```python
from build123d import *

# Parameters (mm, degrees)
SKETCH1_R           = 1.499997
SKETCH1_R_2         = 5.08
BOSS_EXTRUDE1_DEPTH = 13.97
CUT_EXTRUDE1_DEPTH  = 3
FILLET1_R           = 1.27
SKETCH3_R           = 3.302
CUT_EXTRUDE2_DEPTH  = 41.275
CUT_EXTRUDE3_DEPTH  = 5.842
BOSS_EXTRUDE2_DEPTH = 25.4
FILLET2_R           = 2.54


with BuildPart() as part:
    # Sketch1 → Boss-Extrude1 (new body)
    with BuildSketch(Plane.XY):
        Polygon((-12.7, 33.2994), (-5.715, 33.2994), (-5.715, 39.6494), (5.715, 39.6494), (5.715, 33.2994), (28.575, 33.2994), (28.575, -33.2994), (5.715, -33.2994), (5.715, -39.6494), (-5.715, -39.6494), (-5.715, -33.2994), (-12.7, -33.2994), align=None)
        with Locations((0, 8.001)):
            Circle(SKETCH1_R, mode=Mode.SUBTRACT)
        with Locations((8.001, 0)):
            Circle(SKETCH1_R, mode=Mode.SUBTRACT)
        Circle(SKETCH1_R_2, mode=Mode.SUBTRACT)
        with Locations((0, -8.001)):
            Circle(SKETCH1_R, mode=Mode.SUBTRACT)
        with Locations((-8.001, 0)):
            Circle(SKETCH1_R, mode=Mode.SUBTRACT)
    extrude(amount=BOSS_EXTRUDE1_DEPTH)

    # Sketch2 → Cut-Extrude1 (cut)
    with BuildSketch(Plane(origin=(0, 0, 0), x_dir=(-1, 0, 0), z_dir=(0, 0, -1))):
        Polygon((8.001, -3.579571669), (11.101, -1.789785834), (11.101, 1.789785834), (8.001, 3.579571669), (4.901, 1.789785834), (4.901, -1.789785834), align=None)
        Polygon((3.579571669, 8.001), (1.789785834, 11.101), (-1.789785834, 11.101), (-3.579571669, 8.001), (-1.789785834, 4.901), (1.789785834, 4.901), align=None)
        Polygon((-3.579571669, -8.001), (-1.789785834, -11.101), (1.789785834, -11.101), (3.579571669, -8.001), (1.789785834, -4.901), (-1.789785834, -4.901), align=None)
        Polygon((-8.001, 3.579571669), (-11.101, 1.789785834), (-11.101, -1.789785834), (-8.001, -3.579571669), (-4.901, -1.789785834), (-4.901, 1.789785834), align=None)
    extrude(amount=-CUT_EXTRUDE1_DEPTH, mode=Mode.SUBTRACT)

    # Fillet1
    # the kernel refuses this fillet: 1.27 mm, written as the material it takes off along each edge
    with BuildSketch(Plane(origin=(-4.901, -1.336637198, 3), x_dir=(0.3505491054701989, -0.9365443527425935, 0), z_dir=(0, 0, -1)), Plane(origin=(-1.336637198, 4.901, 3), x_dir=(-0.9365443527425947, -0.3505491054701953, 0), z_dir=(0, 0, -1)), Plane(origin=(1.336637198, -4.901, 3), x_dir=(0.9365443527425922, 0.3505491054702024, 0), z_dir=(0, 0, -1))) as fillet1_piece_1:
        with BuildLine():
            CenterArc((1.048997579, 1.264640212), FILLET1_R, 240.540119445, 24.194103812)
            Line((0.424393796, 0.158850849), (0, 0))
            ThreePointArc((0, 0), (0.466221146, 0.021439153), (0.932442292, 0))
        make_face()
    extrude(amount=5.331105731, mode=Mode.SUBTRACT)
    with BuildSketch(Plane(origin=(-4.901, 1.336637198, 3), x_dir=(0.35054910547019297, 0.9365443527425957, 0), z_dir=(0, 0, -1)), Plane(origin=(1.336637198, 4.901, 3), x_dir=(0.9365443527425946, -0.3505491054701959, 0), z_dir=(0, 0, -1)), Plane(origin=(-1.336637198, -4.901, 3), x_dir=(-0.9365443527425968, 0.35054910547018975, 0), z_dir=(0, 0, -1))) as fillet1_piece_2:
        with BuildLine():
            CenterArc((1.048997579, -1.264640212), FILLET1_R, 95.265776743, 24.194103812)
            Line((0.424393796, -0.158850849), (0, 0))
            ThreePointArc((0, 0), (0.466221146, -0.021439153), (0.932442292, 0))
        make_face()
    extrude(amount=5.331105731, mode=Mode.SUBTRACT)
    with BuildSketch(Plane(origin=(4.901, 1.336637198, 3), x_dir=(0, 1, 0), z_dir=(0, 0, -1))) as fillet1_piece_3:
        with BuildLine():
            CenterArc((1.425751253, 0.816666486), FILLET1_R, 220.019214916, 24.194103812)
            ThreePointArc((0.873273563, -0.326866811), (0.444152257, -0.143354688), (0, 0))
            Line((0, 0), (0.453148636, 0))
        make_face()
    extrude(amount=5.331105731, mode=Mode.SUBTRACT)
    with BuildSketch(Plane(origin=(4.901, -1.336637198, 3), x_dir=(0, -1, 0), z_dir=(0, 0, -1))) as fillet1_piece_4:
        with BuildLine():
            CenterArc((1.425751253, -0.816666486), FILLET1_R, 115.786681272, 24.194103812)
            ThreePointArc((0.873273563, 0.326866811), (0.444152257, 0.143354688), (0, 0))
            Line((0, 0), (0.453148636, 0))
        make_face()
    extrude(amount=5.331105731, mode=Mode.SUBTRACT)

    # Sketch3 → Cut-Extrude2 (cut)
    with BuildSketch(Plane(origin=(28.575, 0, 0), x_dir=(0, 0, -1), z_dir=(1, 0, 0))):
        with Locations((-6.985, 15.875)):
            Circle(SKETCH3_R)
        with Locations(Location((-6.985, -15.875, 0), (0, 0, 90))):
            Circle(SKETCH3_R)
    extrude(amount=-CUT_EXTRUDE2_DEPTH, mode=Mode.SUBTRACT)

    # Sketch4 → Cut-Extrude3 (cut)
    with BuildSketch(Plane.ZY.offset(12.7)):
        Polygon((12.7, -19.174556788), (6.985, -22.474113577), (1.27, -19.174556788), (1.27, -12.575443212), (6.985, -9.275886423), (12.7, -12.575443212), align=None)
        Polygon((6.985, 22.474113577), (1.27, 19.174556788), (1.27, 12.575443212), (6.985, 9.275886423), (12.7, 12.575443212), (12.7, 19.174556788), align=None)
    extrude(amount=-CUT_EXTRUDE3_DEPTH, mode=Mode.SUBTRACT)

    # Sketch5 → Boss-Extrude2 (add)
    with BuildSketch(Plane(origin=(0, 0, 0), x_dir=(-1, 0, 0), z_dir=(0, 0, -1))):
        Polygon((-28.575, 20.5994), (12.7, 20.5994), (12.7, 33.2994), (5.715, 33.2994), (5.715, 39.6494), (-5.715, 39.6494), (-5.715, 33.2994), (-28.575, 33.2994), align=None)
        Polygon((12.7, -20.5994), (-28.575, -20.5994), (-28.575, -33.2994), (-5.715, -33.2994), (-5.715, -39.6494), (5.715, -39.6494), (5.715, -33.2994), (12.7, -33.2994), align=None)
    extrude(amount=BOSS_EXTRUDE2_DEPTH)

    # Fillet2
    fillet2_edges = [part.edges().sort_by_distance(p)[0] for p in [
        (7.9375, -20.5994, 0),
        (7.9375, 20.5994, 0),
    ]]
    fillet(fillet2_edges, radius=FILLET2_R)


solid = part.part
```
For this review, take the finished solid that the model builds, in its own axes (mm). A direction names the side the tool comes from. Give positions to 0.01 mm unless a question says otherwise; leave off trailing zeros. Write each loop counter-clockwise with the first axis right and the second up, starting at its lowest first coordinate (ties: lowest second). Pieces come first, ordered by that corner, then holes. Notation, with made-up numbers: M 4,21.25 L 34,21.25 A25 cw 34,40.25 Z; hole C 41,-17 d6. An arc over 180 degrees is marked long. One line per item, written item: value.
1) For P1, Ø1.9, axis at y = 38, z = -1.5, coming from the -X side (3 decimals); P2, Ø3, axis at x = -8.5, y = 16.5, coming from the -Z side; P3, Ø2, axis at x = -1, y = 8.5, coming from the -Z side; P4, Ø1.8, axis at x = -8.001, y = 0, coming from the +Z side, all flat-tipped, find the tip position at first contact; note any pin that passes through.
Results are:
P1: stops at x = -5.715
P2: stops at z = 0
P3: stops at z = 3
P4: passes through
2) Take a section at A-A, the plane y = 0. Write out the cut boundary in (x, z) (3 decimals).
Results are:
outline: M -12.7,0 L -11.101,0 L -11.101,3 L -9.501,3 L -9.501,13.97 L -12.7,13.97 Z; M -6.501,3 L -5.08,3 L -5.08,13.97 L -6.501,13.97 Z; M 5.08,3 L 6.501,3 L 6.501,13.97 L 5.08,13.97 Z; M 9.501,3 L 11.101,3 L 11.101,0 L 28.575,0 L 28.575,13.97 L 9.501,13.97 Z
3) Take a section at C-C, the plane z = -14.5. Write out the cut boundary in (x, y) (3 decimals), then the cut area to 3 significant figures.
Results are:
outline: M -12.7,-33.299 L -5.715,-33.299 L -5.715,-39.649 L 5.715,-39.649 L 5.715,-33.299 L 28.575,-33.299 L 28.575,-20.599 L -12.7,-20.599 Z; M -12.7,20.599 L 28.575,20.599 L 28.575,33.299 L 5.715,33.299 L 5.715,39.649 L -5.715,39.649 L -5.715,33.299 L -12.7,33.299 Z
area: 1,190 mm²
4) For faces 1 (the flat face through (-10, -11, 4)), 2 (the flat face through (9.573, -2.672, 1.479)), 3 (the flat face through (-5.715, 36, -5)), list the 3-axis set-ups (+Z, -Z, +X, -X, +Y, -Y) from which the entire face can be reached by the end or side of a thin tool; tool diameter is ignored.
Results are:
face 1: -X
face 2: -Z
face 3: +Z, -Z, -X, +Y
5) For line 1 (Y direction, x = 26.5, z = 7); line 2 (Y direction, x = 0, z = 11.75); line 3 (Z direction, x = -7, y = -13), list the stretches that pass through material, from the lowest coordinate up. Write a range as from..to.
Results are:
line 1: y = -33.3..-19.18, -12.57..12.57, 19.18..33.3
line 2: y = -39.65..-9.5, -6.5..-5.08, 5.08..6.5, 9.5..39.65
line 3: z = 0..1.27, 12.7..13.97
6) Take a section at B-B, the plane x = 0. Write out the cut boundary in (y, z) (3 decimals), then the cut area to 3 significant figures.
Results are:
outline: M -39.649,-25.4 L -20.599,-25.4 L -20.599,-2.54 A2.54 cw -18.059,0 L -11.101,0 L -11.101,3 L -9.501,3 L -9.501,13.97 L -39.649,13.97 Z; M -6.501,3 L -5.08,3 L -5.08,13.97 L -6.501,13.97 Z; M 5.08,3 L 6.501,3 L 6.501,13.97 L 5.08,13.97 Z; M 9.501,3 L 11.101,3 L 11.101,0 L 18.059,0 A2.54 cw 20.599,-2.54 L 20.599,-25.4 L 39.649,-25.4 L 39.649,13.97 L 9.501,13.97 Z; hole C -15.875,6.985 d6.604; hole C 15.875,6.985 d6.604
area: 1,770 mm²
7) Take a section at D-D, the plane z = 9. Count the separate pieces of the cut face and the enclosed holes in it, then the cut area to 3 significant figures.
Results are:
separate pieces: 3
enclosed holes: 5
area: 2,290 mm²
8) The part is to be moulded in two halves that separate along Y. For faces 4 (the flat face through (13, 1, 13.97)), 5 (the flat face through (-9.529, -2.697, 1.479)), say which applies: +Y half, -Y half, draft (parallel to the pull), parting line (faces both ways), or undercut.
Results are:
face 4: draft
face 5: undercut
